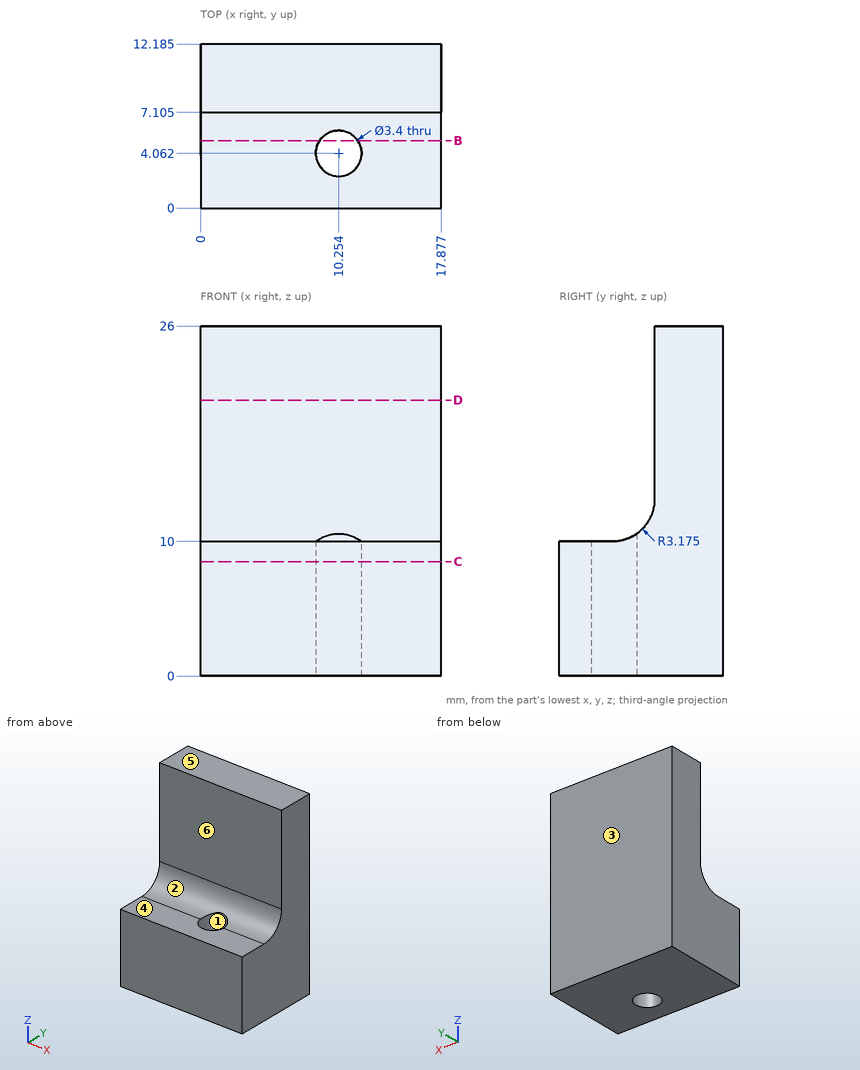
Could you check a few things on this drawing? It's one solid part, dimensions in mm from its lowest x, y, z. A direction names the side the tool comes from. Give positions to 0.01 mm unless a question says otherwise; leave off trailing zeros. Order: outer loops, then holes, each group sorted by start corner. A loop starts at its lowest first (then second) coordinate and runs counter-clockwise, first axis right, second up.
1. For pin 1 (10 mm diameter, centred on x = 13.5, z = 16, fed in from -Y); pin 2 (2 mm diameter, centred on x = 10.25, y = 4.06, fed in from -Z); pin 3 (2 mm diameter, centred on x = 10, y = 2, fed in from +Z), each with a flat end and sliding along its axis, tell me the tip position at first contact or that it passes through.
Answers below:
pin 1: stops at y = 6.24
pin 2: passes through
pin 3: stops at z = 10
2. Suppose I cut it at D-D (z = 20.5). Write out the boundary of the cut face in (x, y) (1 decimal).
Answers below:
outline: (0, 7.1) - (17.9, 7.1) - (17.9, 12.2) - (0, 12.2) - close
3. Which directions (+Z, -Z, +X, -X, +Y, -Y) give clear straight access to the entire face, cutting with the end or side of a thin tool? Please do the marked faces 5 and 6.
Answers below:
face 5: +Z, +X, -X, +Y, -Y
face 6: +Z, +X, -X, -Y
4. Suppose I cut it at C-C (z = 8.5). Write out the boundary of the cut face in (x, y) (1 decimal).
Answers below:
outline: (0, 0) - (17.9, 0) - (17.9, 12.2) - (0, 12.2) - close; hole circle Ø3.4 at (10.3, 4.1)
5. I need wall thicknesses on L1, parallel to Z at x = 4.5, y = 3.25; L2, parallel to Y at x = 10.5, z = 2 (1 decimal); L3, parallel to Y at x = 13.75, z = 14.75 (1 decimal). Which ranges of each line are inside material? Lowest first, please.
Answers below:
L1: z = 0 to 10
L2: y = 0 to 2.4, 5.7 to 12.2
L3: y = 7.1 to 12.2
6. Suppose I cut it at B-B (y = 5). Write out the boundary of the cut face in (x, z) (1 decimal).
Answers below:
outline: (0, 0) - (8.8, 0) - (8.8, 10.2) - (0, 10.2) - close; (11.7, 0) - (17.9, 0) - (17.9, 10.2) - (11.7, 10.2) - close
7. Thinking about a two-plate mould opening in Y: for the marked faces 1, 2, 3 and 4, which applies, +Y half, -Y half, draft (parallel to the pull), parting line (faces both ways), or undercut?
Answers below:
face 1: undercut
face 2: -Y half
face 3: +Y half
face 4: draft
